Part print with two shaded views. Sizes in mm from the minimum x, y, z corner. A direction names the side the tool comes from. Round coordinates to 2 decimals unless told otherwise and drop trailing zeros. Write each loop counter-clockwise with the first axis right and the second up, starting at its lowest first coordinate (ties: lowest second). Pieces come first, ordered by that corner, then holes. Notation, with made-up numbers: (63.5, 4) -> (88.5, 4) arc R33 ccw to (88.5, 38) -> close; hole circle Ø2 at (-35, 74). An arc over 180 degrees is marked (long way). Answer in a Markdown table with one row per item.
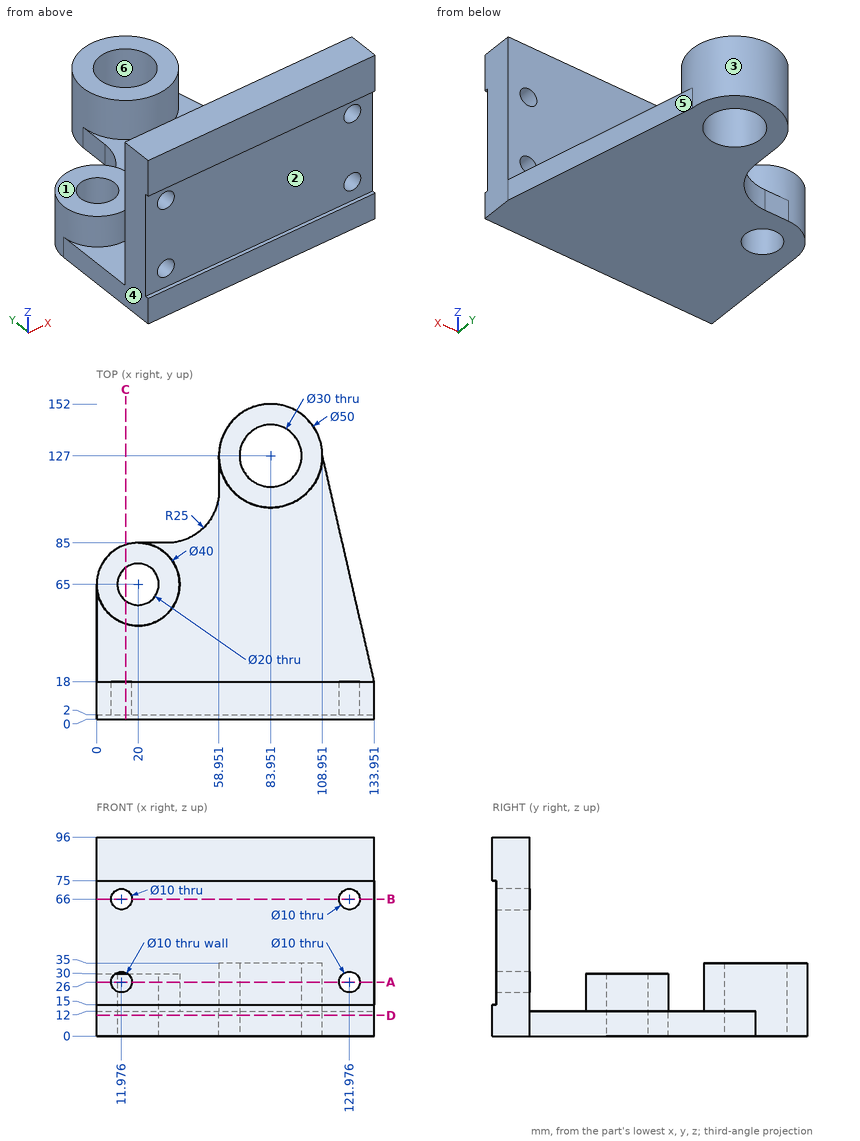
Q1. Saw through at D-D on z = 10. Write the cut outline in (x, y).
A:
| item | result |
|---|---|
| outline | (0, 0) -> (133.95, 0) -> (133.95, 18) -> (108.95, 127) arc R25 ccw to (58.95, 127) -> (58.95, 110) arc R25 cw to (33.95, 85) -> (20, 85) arc R20 ccw to (0, 65) -> close; hole circle Ø20 at (20, 65); hole circle Ø30 at (83.95, 127) |
Q2. Wall check: line 1 (X direction, y = 13, z = 66) (1 decimal); line 2 (Y direction, x = 19.5, z = 20); line 3 (Y direction, x = 70.5, z = 13.5) (1 decimal). Give the ranges that are in metal, low to high. Write a range as [from, to].
A:
| item | result |
|---|---|
| line 1 | [0, 7], [17, 117], [127, 134] |
| line 2 | [2, 18], [45.01, 55.01], [74.99, 84.99] |
| line 3 | [0, 18], [105.9, 120.4], [133.6, 148.1] |
Q3. Which spindle directions (+Z, -Z, +X, -X, +Y, -Y) get a long thin tool onto all of the face, cutting with end or side? Do the marked faces 1, 2 and 3. Say none if no direction does.
A:
| item | result |
|---|---|
| face 1 | +Z, +X, -X, +Y |
| face 2 | +X, -X, -Y |
| face 3 | +Z |
Q4. Drop flat-ended pins along their axis: P1, Ø10, axis at y = 64, z = 16.5, coming from the +X side; P2, Ø9, axis at x = 11.98, z = 26, coming from the +Y side; P3, Ø3, axis at x = 115.5, z = 69.5, coming from the -Y side; P4, Ø9, axis at x = 121.98, z = 66, coming from the -Y side. Give the stop position or say it passes through.
A:
| item | result |
|---|---|
| P1 | x = 123.9 |
| P2 | y = 84.69 |
| P3 | y = 2 |
| P4 | through |
Q5. Saw through at B-B on z = 66. Write the cut outline in (x, y) (1 decimal), plus the area to 3 significant figures.
A:
| item | result |
|---|---|
| outline | (0, 2) -> (7, 2) -> (7, 18) -> (0, 18) -> close; (17, 2) -> (117, 2) -> (117, 18) -> (17, 18) -> close; (127, 2) -> (134, 2) -> (134, 18) -> (127, 18) -> close |
| area | 1,820 mm² |
Q6. Saw through at C-C on x = 14. Write the cut outline in (y, z).
A:
| item | result |
|---|---|
| outline | (0, 0) -> (57, 0) -> (57, 30) -> (45.92, 30) -> (45.92, 12) -> (18, 12) -> (18, 21.43) -> (2, 21.43) -> (2, 15) -> (0, 15) -> close; (0, 75) -> (2, 75) -> (2, 70.57) -> (18, 70.57) -> (18, 96) -> (0, 96) -> close; (2, 30.57) -> (18, 30.57) -> (18, 61.43) -> (2, 61.43) -> close; (73, 0) -> (84.08, 0) -> (84.08, 30) -> (73, 30) -> close |
Q7. Saw through at A-A on z = 26. Write the cut outline in (x, y) (1 decimal), plus the area to 3 significant figures.
A:
| item | result |
|---|---|
| outline | (0, 2) -> (7, 2) -> (7, 18) -> (0, 18) -> close; circle Ø40 at (20, 65); (17, 2) -> (117, 2) -> (117, 18) -> (17, 18) -> close; circle Ø50 at (84, 127); (127, 2) -> (134, 2) -> (134, 18) -> (127, 18) -> close; hole circle Ø20 at (20, 65); hole circle Ø30 at (84, 127) |
| area | 4,020 mm² |
Q8. Two-plate mould, pull along X, no slides. Class the marked faces 4, 5 and 6: released by +X, released by -X, zero draft, split by the parting line, or undercut.
A:
| item | result |
|---|---|
| face 4 | released by -X |
| face 5 | released by +X |
| face 6 | undercut |
